Geometry: final body of the model. Coordinates: model frame, mm. Face numbers are marked on the shaded views. A direction names the side the tool comes from. Round coordinates to 2 decimals unless told otherwise and drop trailing zeros. Loops run counter-clockwise (first coordinate to the right, second up) from the corner with the lowest first, then second, coordinate; pieces in that order, holes last. Notation, with made-up numbers: (-8.75, 6) - (19.25, 6) arc R25 cw to (19.25, 18) - close; hole circle Ø3 at (-26.5, -28.5). An arc over 180 degrees is marked (long way). Return JSON: item names as keys, results as strings. Group by question number.
1. Section C-C on y = 100. Return loops of the section in (x, z).
2. Set-up query: the marked faces 4 and 5. Return all of +Z, -Z, +X, -X, +Y, -Y with unobstructed straight access to the full face (end or side cutting, diameter ignored); none if empty.
3. Section A-A on x = 102. Return loops of the section in (y, z), and give its area (3 significant figures).
4. First-contact query: pin 1 Ø2 at (x, y) = (-73.5, -89.5) entering from +Z (3 decimals). Flat tip, straight axial feed; report the tip coordinate or a pass-through.
5. Section B-B on z = 1171. Return loops of the section in (x, y).
6. Material intervals for probe 1 along X at (y, z) = (180.5, 1156); probe 2 along X at (y, z) = (-101.5, 1176.5), sorted ascending.
7. Section D-D on y = 170.5. Return loops of the section in (x, z), and give its area (3 significant figures).
8. Draft query along X for the marked faces 1, 2 and 3. Return one class per face: +X half, -X half, draft (parallel to the pull), parting line (faces both ways), or undercut.
from build123d import *

# Parameters (mm, degrees)
ESQUISSE1_W              = 400
ESQUISSE1_H              = 400
BOSS_EXTRU_1_DEPTH       = 1200
ESQUISSE4_W              = 400
ESQUISSE4_H              = 130.6
ENL_V_MAT_EXTRU_1_DEPTH  = 300
ENL_V_MAT_EXTRU_2_DEPTH  = 100
ESQUISSE13_W             = 400
ESQUISSE13_H             = 400
ENL_V_MAT_EXTRU_10_DEPTH = 400
ENL_V_START              = -35
ENL_V_MAT_EXTRU_11_DEPTH = 400
CONG_3_R                 = 10
ENL_V_MAT_EXTRU_12_DEPTH = 100
CONG_5_R                 = 5
COQUE1_START             = -90
COQUE1_OUTLINE_W         = 380
COQUE1_OUTLINE_H         = 591.664973081
COQUE1_DEPTH             = 280
COQUE1_START_2           = -190
COQUE1_2_DEPTH           = 345.26524617
COQUE1_3_OUTLINE_W       = 380
COQUE1_3_OUTLINE_H       = 150.6
COQUE1_3_DEPTH           = 80
COQUE1_4_DEPTH           = 380
COQUE1_START_3           = 175
COQUE1_5_DEPTH           = 15
ESQUISSE21_W             = 360
ESQUISSE21_H             = 260
ENL_V_MAT_EXTRU_13_DEPTH = 300
ENL_V_MAT_EXTRU_14_DEPTH = 674.894679675
ENL_V_MAT_EXTRU_15_DEPTH = 280
ESQUISSE24_W             = 400
ESQUISSE24_H             = 742.264973081
ENL_V_MAT_EXTRU_16_DEPTH = 1281.624847487
BOSS_EXTRU_2_REACH       = 1257.428
ESQUISSE25_W             = 380
ESQUISSE25_H             = 10


with BuildPart() as part:
    # Esquisse1 → Boss.-Extru.1 (new body)
    with BuildSketch(Plane.XY):
        Rectangle(ESQUISSE1_W, ESQUISSE1_H)
    extrude(amount=BOSS_EXTRU_1_DEPTH)

    # Esquisse4 → Enlèv. mat.-Extru.1 (cut)
    with BuildSketch(Plane(origin=(0, 200, 0), x_dir=(1, 0, 0), z_dir=(0, 1, 0))):
        with Locations((0, -1076.964973081)):
            Rectangle(ESQUISSE4_W, ESQUISSE4_H)
    extrude(amount=-ENL_V_MAT_EXTRU_1_DEPTH, mode=Mode.SUBTRACT)

    # Esquisse5 → Enlèv. mat.-Extru.2 (cut)
    with BuildSketch(Plane.XZ.offset(200)):
        with BuildLine():
            Line((-145, 902.264973081), (145, 902.264973081))
            ThreePointArc((145, 902.264973081), (155.606601718, 897.871574799), (160, 887.264973081))
            Line((160, 887.264973081), (160, 797.264973081))
            ThreePointArc((160, 797.264973081), (155.606601718, 786.658371363), (145, 782.264973081))
            Line((145, 782.264973081), (-145, 782.264973081))
            ThreePointArc((-145, 782.264973081), (-155.606601718, 786.658371363), (-160, 797.264973081))
            Line((-160, 797.264973081), (-160, 887.264973081))
            ThreePointArc((-160, 887.264973081), (-155.606601718, 897.871574799), (-145, 902.264973081))
        make_face()
    extrude(amount=-ENL_V_MAT_EXTRU_2_DEPTH, mode=Mode.SUBTRACT)

    # Esquisse13 → Enlèv. mat.-Extru.10 (cut)
    with BuildSketch(Plane(origin=(0, 0, 0), x_dir=(-1, 0, 0), z_dir=(0, 0, -1))):
        Rectangle(ESQUISSE13_W, ESQUISSE13_H)
    extrude(amount=-ENL_V_MAT_EXTRU_10_DEPTH, mode=Mode.SUBTRACT)

    # Esquisse18 → Enlèv. mat.-Extru.11 (cut)
    with BuildSketch(Plane(origin=(200, 0, 0), x_dir=(0, 0, -1), z_dir=(1, 0, 0)).offset(ENL_V_START)):
        with BuildLine():
            Line((-1142.264973081, 200), (-1176.793054109, 200))
            ThreePointArc((-1176.793054109, 200), (-1165.318675352, 175.963910431), (-1142.264973081, 162.625178063))
            Line((-1142.264973081, 162.625178063), (-1142.264973081, 200))
        make_face()
    extrude(amount=-ENL_V_MAT_EXTRU_11_DEPTH, mode=Mode.SUBTRACT)

    # Congé3
    cong_3_edges = [part.edges().sort_by_distance(p)[0] for p in [
        (-17.5, 162.625178063, 1142.264973081),
    ]]
    fillet(cong_3_edges, radius=CONG_3_R)

    # Esquisse20 → Enlèv. mat.-Extru.12 (cut)
    with BuildSketch(Plane.XZ.offset(200)):
        with BuildLine():
            Line((155, 703.393343593), (-155, 703.393343593))
            ThreePointArc((-155, 703.393343593), (-169.142135624, 697.535479217), (-175, 683.393343593))
            Line((-175, 683.393343593), (-175, 400))
            Line((-175, 400), (175, 400))
            Line((175, 400), (175, 683.393343593))
            ThreePointArc((175, 683.393343593), (169.142135624, 697.535479217), (155, 703.393343593))
        make_face()
    extrude(amount=-ENL_V_MAT_EXTRU_12_DEPTH, mode=Mode.SUBTRACT)

    # Congé5
    cong_5_edges = [part.edges().sort_by_distance(p)[0] for p in [
        (0, -100, 400),
        (175, -150, 400),
        (-175, -150, 400),
    ]]
    fillet(cong_5_edges, radius=CONG_5_R)

    # Coque1: read off the stored shape, not the designer's step
    # Coque1 outline → Coque1 (cut)
    with BuildSketch(Plane(origin=(0, 0, 0), x_dir=(1, 0, 0), z_dir=(0, 1, 0)).offset(COQUE1_START)):
        with Locations((0, -705.83248654)):
            Rectangle(COQUE1_OUTLINE_W, COQUE1_OUTLINE_H)
    extrude(amount=COQUE1_DEPTH, mode=Mode.SUBTRACT)

    # Coque1 2 outline → Coque1 2 (cut)
    # profile 1 of 2: a face of its own
    with BuildSketch(Plane(origin=(0, 0, 0), x_dir=(1, 0, 0), z_dir=(0, 1, 0)).offset(COQUE1_START_2)):
        with BuildLine():
            Line((190, -1001.664973081), (190, -410))
            Line((190, -410), (185, -410))
            Line((185, -410), (185, -683.393343593))
            ThreePointArc((185, -683.393343593), (176.213203435, -704.606547029), (155, -713.393343593))
            Line((155, -713.393343593), (-155, -713.393343593))
            ThreePointArc((-155, -713.393343593), (-176.213203435, -704.606547029), (-185, -683.393343593))
            Line((-185, -683.393343593), (-185, -410))
            Line((-185, -410), (-190, -410))
            Line((-190, -410), (-190, -1001.664973081))
            Line((-190, -1001.664973081), (190, -1001.664973081))
        make_face()
        with BuildLine():
            Line((-170, -887.264973081), (-170, -797.264973081))
            ThreePointArc((-170, -797.264973081), (-162.67766953, -779.587303551), (-145, -772.264973081))
            Line((-145, -772.264973081), (145, -772.264973081))
            ThreePointArc((145, -772.264973081), (162.67766953, -779.587303551), (170, -797.264973081))
            Line((170, -797.264973081), (170, -887.264973081))
            ThreePointArc((170, -887.264973081), (162.67766953, -904.942642611), (145, -912.264973081))
            Line((145, -912.264973081), (-145, -912.264973081))
            ThreePointArc((-145, -912.264973081), (-162.67766953, -904.942642611), (-170, -887.264973081))
        make_face(mode=Mode.SUBTRACT)
    # profile 2 of 2: a face of its own
    with BuildSketch(Plane(origin=(0, 0, 0), x_dir=(1, 0, 0), z_dir=(0, 1, 0)).offset(COQUE1_START_2)):
        Polygon((190, -1200), (190, -1152.264973081), (175, -1152.264973081), (-190, -1152.264973081), (-190, -1200), align=None)
    extrude(amount=COQUE1_2_DEPTH, mode=Mode.SUBTRACT)

    # Coque1 3 outline → Coque1 3 (cut)
    with BuildSketch(Plane(origin=(0, 0, 0), x_dir=(1, 0, 0), z_dir=(0, 1, 0)).offset(COQUE1_START_2)):
        with Locations((0, -1076.964973081)):
            Rectangle(COQUE1_3_OUTLINE_W, COQUE1_3_OUTLINE_H)
    extrude(amount=COQUE1_3_DEPTH, mode=Mode.SUBTRACT)

    # Coque1 4 outline → Coque1 4 (cut)
    with BuildSketch(Plane.YZ.offset(COQUE1_START_2)):
        with BuildLine():
            Line((190, 1184.731629159), (190, 1200))
            Line((190, 1200), (155.26524617, 1200))
            Line((155.26524617, 1200), (155.26524617, 1152.264973081))
            ThreePointArc((155.26524617, 1152.264973081), (168.943107712, 1172.445563441), (190, 1184.731629159))
        make_face()
    extrude(amount=COQUE1_4_DEPTH, mode=Mode.SUBTRACT)

    # Coque1 5 outline → Coque1 5 (cut)
    with BuildSketch(Plane.YZ.offset(COQUE1_START_3)):
        with BuildLine():
            Line((190, 1152.264973081), (190, 1184.731629159))
            ThreePointArc((190, 1184.731629159), (168.943107712, 1172.445563441), (155.26524617, 1152.264973081))
            Line((155.26524617, 1152.264973081), (190, 1152.264973081))
        make_face()
    extrude(amount=COQUE1_5_DEPTH, mode=Mode.SUBTRACT)

    # Esquisse21 → Enlèv. mat.-Extru.13 (cut)
    with BuildSketch(Plane.XY.offset(1011.664973081)):
        with Locations((0, 50)):
            Rectangle(ESQUISSE21_W, ESQUISSE21_H)
    extrude(amount=-ENL_V_MAT_EXTRU_13_DEPTH, mode=Mode.SUBTRACT)

    # Esquisse22 → Enlèv. mat.-Extru.14 (cut, through all)
    with BuildSketch(Plane.XY.offset(1011.664973081)):
        Polygon((-180, 180), (180, 180), (200, 180), (200, 200), (-200, 200), (-200, 180), align=None)
    extrude(amount=-ENL_V_MAT_EXTRU_14_DEPTH, mode=Mode.SUBTRACT)

    # Esquisse23 → Enlèv. mat.-Extru.15 (cut)
    with BuildSketch(Plane(origin=(0, 180, 0), x_dir=(1, 0, 0), z_dir=(0, 1, 0))):
        Polygon((-200, -410), (-190, -410), (190, -410), (200, -410), (200, -400), (-200, -400), align=None)
    extrude(amount=-ENL_V_MAT_EXTRU_15_DEPTH, mode=Mode.SUBTRACT)

    # Esquisse24 → Enlèv. mat.-Extru.16 (cut, through all)
    with BuildSketch(Plane.XZ.offset(200)):
        with Locations((0, 771.132486541)):
            Rectangle(ESQUISSE24_W, ESQUISSE24_H)
    extrude(amount=-ENL_V_MAT_EXTRU_16_DEPTH, mode=Mode.SUBTRACT)

    # Esquisse25 → Boss.-Extru.2 (add, up to next)
    with BuildSketch(Plane.XZ.offset(110), mode=Mode.PRIVATE) as boss_extru_2_sk1:
        with Locations((0, 1147.264973081)):
            Rectangle(ESQUISSE25_W, ESQUISSE25_H)
    boss_extru_2_tool1 = extrude(boss_extru_2_sk1.sketch, amount=BOSS_EXTRU_2_REACH, mode=Mode.PRIVATE) - part.part
    add(boss_extru_2_tool1.solids().sort_by_distance((0, -110, 1147.264973))[0])


solid = part.part
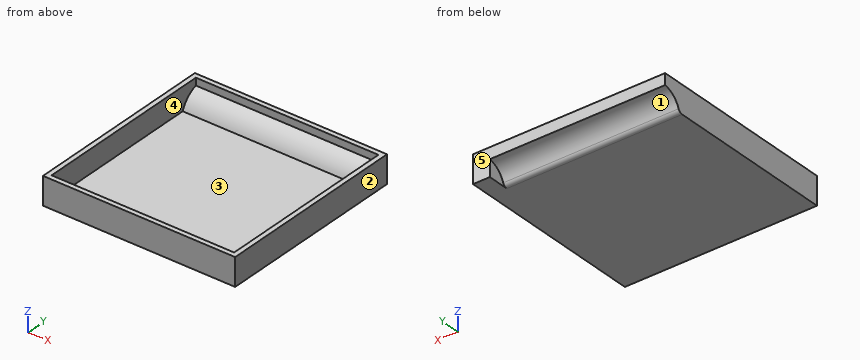
Taken from the geometry:
{
 "1": {"outline": "(-200, 1142.26) - (200, 1142.26) - (200, 1200) - (190, 1200) - (190, 1152.26) - (-190, 1152.26) - (-190, 1200) - (-200, 1200) - close"},
 "2": {"face 4": "+Z", "face 5": "+Z, -Z, +X, -X, +Y"},
 "3": {"outline": "(-200, 1142.26) - (155.27, 1142.26) arc R10 ccw to (164.58, 1148.63) arc R45 cw to (200, 1176.79) - (200, 1200) - (190, 1200) - (190, 1184.73) arc R55 ccw to (155.27, 1152.26) - (-190, 1152.26) - (-190, 1200) - (-200, 1200) - close", "area": "4,760 mm2"},
 "4": {"pin 1": "z = 1152.265"},
 "5": {"outline": "(-200, -200) - (200, -200) - (200, 200) - (165, 200) - (165, 183.6) - (-200, 183.6) - close; hole (-190, -190) - (190, -190) - (190, 190) - (175, 190) - (175, 167.45) - (-190, 167.45) - close"},
 "6": {"probe 1": "165 to 175, 190 to 200", "probe 2": "-200 to -190, 190 to 200"},
 "7": {"outline": "(-200, 1159.26) - (165, 1159.26) - (165, 1142.26) - (200, 1142.26) - (200, 1200) - (190, 1200) - (190, 1152.26) - (175, 1152.26) - (175, 1173.85) - (-190, 1173.85) - (-190, 1200) - (-200, 1200) - close", "area": "6,630 mm2"},
 "8": {"face 1": "draft", "face 2": "+X half", "face 3": "undercut"}
}
